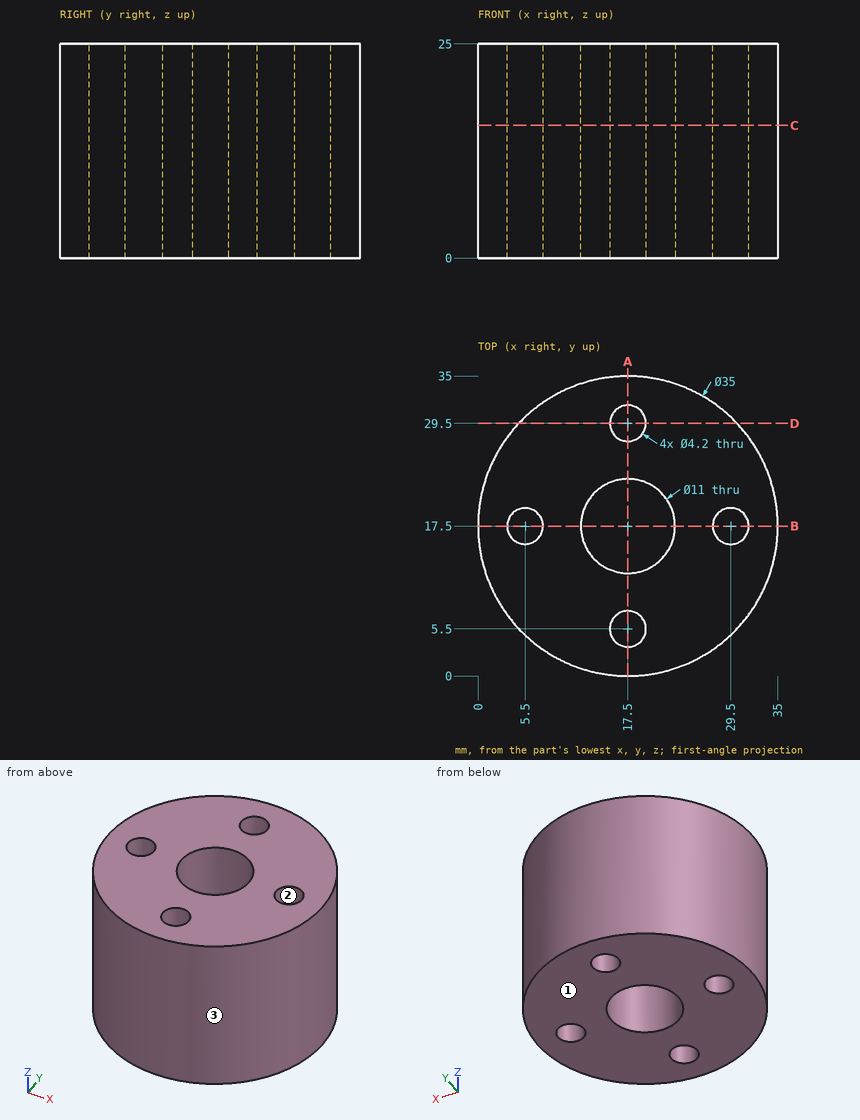
The figure shows three views and two pictorial views of one solid part (mm, origin at its lowest corner). Answer the questions. Give positions to 0.01 mm unless a question says otherwise; leave off trailing zeros. Order: outer loops, then holes, each group sorted by start corner. A loop starts at its lowest first (then second) coordinate and runs counter-clockwise, first axis right, second up. Notation, with made-up numbers: (42.25, 31) -> (61.25, 31) arc R23 ccw to (61.25, 60) -> close; hole circle Ø3 at (89.25, 29.5). An arc over 180 degrees is marked (long way). Answer as a JSON object with one key per item and string values. Group by question number.
Item 1: Flat-ended cylindrical pins translate along their axes: pin 1 (12 mm diameter, centred on x = 5.5, z = 15, fed in from +Y); pin 2 (4 mm diameter, centred on x = 17.5, y = 29.5, fed in from -Z); pin 3 (2 mm diameter, centred on y = 9.5, z = 15.5, fed in from -X); pin 4 (1 mm diameter, centred on x = 8.5, z = 11, fed in from +Y). Find the tip coordinate at first contact, or state that the pin passes through.
Item 2: The part is cut by section C-C on z = 15.5. Write down the section's boundary in (x, y), and give its area (3 significant figures).
Item 3: Consider L1, parallel to Y at x = 17.5, z = 7.5; L2, parallel to Y at x = 16, z = 13.25; L3, parallel to X at y = 14, z = 18.5. Determine where each line is inside the solid, lowest interval first. Write a range as from..to.
Item 4: The part is cut by section D-D on y = 29.5. Write down the section's boundary in (x, z), and give its area (3 significant figures).
Item 5: Determine the mould class of the marked faces 1, 2 and 3 for opening direction X: pulls with the +X half, pulls with the -X half, needs draft (parallel to the pull), parting line crosses it, or undercut.
Item 6: The part is cut by section A-A on x = 17.5. Write down the section's boundary in (y, z), and give its area (3 significant figures).
Result set:
{
 "1": {"pin 1": "y = 33.94", "pin 2": "through", "pin 3": "x = 1.46", "pin 4": "y = 32.8"},
 "2": {"outline": "circle Ø35 at (17.5, 17.5); hole circle Ø4.2 at (5.5, 17.5); hole circle Ø11 at (17.5, 17.5); hole circle Ø4.2 at (17.5, 5.5); hole circle Ø4.2 at (17.5, 29.5); hole circle Ø4.2 at (29.5, 17.5)", "area": "812 mm²"},
 "3": {"L1": "0..3.4, 7.6..12, 23..27.4, 31.6..35", "L2": "0.06..4.03, 6.97..12.21, 22.79..28.03, 30.97..34.94", "L3": "0.35..13.26, 21.74..34.65"},
 "4": {"outline": "(4.76, 0) -> (15.4, 0) -> (15.4, 25) -> (4.76, 25) -> close; (19.6, 0) -> (30.24, 0) -> (30.24, 25) -> (19.6, 25) -> close", "area": "532 mm²"},
 "5": {"face 1": "needs draft", "face 2": "undercut", "face 3": "parting line crosses it"},
 "6": {"outline": "(0, 0) -> (3.4, 0) -> (3.4, 25) -> (0, 25) -> close; (7.6, 0) -> (12, 0) -> (12, 25) -> (7.6, 25) -> close; (23, 0) -> (27.4, 0) -> (27.4, 25) -> (23, 25) -> close; (31.6, 0) -> (35, 0) -> (35, 25) -> (31.6, 25) -> close", "area": "390 mm²"}
}
